Work out the finished part from the listing and answer in its coordinate system (mm). Face numbers are marked on the shaded views. Coordinates: 2 decimals unless noted, no trailing zeros. Order: outer loops, then holes, each group sorted by start corner. A loop starts at its lowest first (then second) coordinate and runs counter-clockwise, first axis right, second up. Notation, with made-up numbers: M 76.5,24 L 92.5,24 A18 ccw 92.5,50 Z; hole C 30.5,-34 d10. An arc over 180 degrees is marked long. Answer in a Markdown table with one row per item. Add a question column.
Item 1: The part is cut by section C-C (y = 1.9). Write down the section's boundary in (x, z).
Item 2: The part is cut by section B-B (x = -2.4). Write down the section's boundary in (y, z), then the cut area to 3 significant figures.
Item 3: Consider line 1 (Y direction, x = 0.1, z = 6.25); line 2 (Y direction, x = -0.85, z = 16.75); line 3 (X direction, y = 0.75, z = 5.75). Determine where each line is inside the solid, lowest interval first. Write a range as from..to.
Item 4: Flat-ended cylindrical pins translate along their axes: pin 1 Ø2 at (x, z) = (2, 13.5) entering from -Y; pin 2 Ø1.5 at (x, y) = (0, 0) entering from -Z; pin 3 Ø1 at (y, z) = (-2, 8) entering from -X. Find the tip coordinate at first contact, or state that the pin passes through.
Item 5: The mould has two halves that part along Y. Classify the marked faces 1, 2, 3 and 4: released by +Y, released by -Y, zero draft, split by the parting line, or undercut.
Item 6: The part is cut by section A-A (z = 4). Write down the section's boundary in (x, y).
Autodesk Inventor part; units mm, degrees
ref_plane "YZ Plane" through (0, 0, 0) normal (1, 0, 0) x (0, 1, 0)
ref_plane "XZ Plane" through (0, 0, 0) normal (0, 1, 0) x (-1, 0, 0)
ref_plane "XY Plane" through (0, 0, 0) normal (0, 0, 1) x (1, 0, 0)
sketch "スケッチ1" plane through (0, 0, 0) normal (0, 0, 1) x (1, 0, 0)
  circle A0 centre (0, 0) radius 3
  dimension "d0" = 6
extrude "押し出し1" add sketch "スケッチ1" along normal blind 20
sketch "スケッチ2" plane through (0, 0, 20) normal (0, 0, 1) x (1, 0, 0)
  point P0 (0, 0)
  point P1 (0, 0)
hole "穴1" at (0, 0, 20) direction (0, 0, -1) diameter 2.459 depth 8.8 tip angle 118
sketch "スケッチ3" plane through (0, 0, 0) normal (0, 0, -1) x (-1, 0, 0)
  circle A0 centre (0, 0) radius 1.2295
hole "穴2" at (0, 0, 0) direction (0, 0, 1) diameter 2.459 depth 8.8 tip angle 118
properties part number "base_part1" material "アルミニウム 6061"
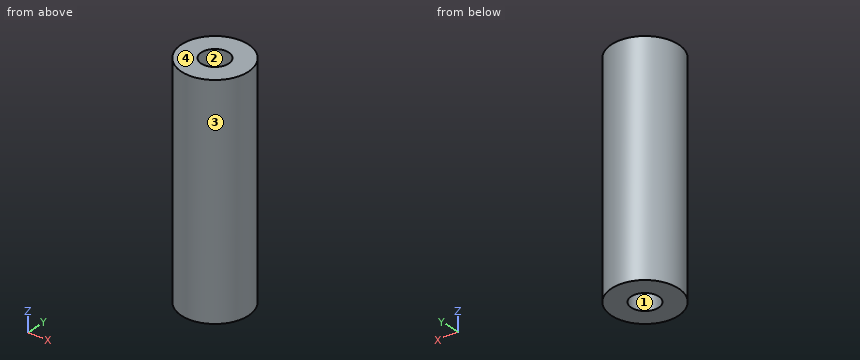
Reply:
| question | item | result |
|---|---|---|
| 1 | outline | M -2.32,0 L 2.32,0 L 2.32,20 L -2.32,20 Z |
| 2 | outline | M -1.8,0 L 1.8,0 L 1.8,20 L -1.8,20 Z |
| 2 | area | 72.0 mm2 |
| 3 | line 1 | y = -3..-1.23, 1.23..3 |
| 3 | line 2 | y = -2.88..-0.89, 0.89..2.88 |
| 3 | line 3 | x = -2.9..-0.97, 0.97..2.9 |
| 4 | pin 1 | stops at y = -2.83 |
| 4 | pin 2 | stops at z = 9.09 |
| 4 | pin 3 | stops at x = -2.6 |
| 5 | face 1 | undercut |
| 5 | face 2 | undercut |
| 5 | face 3 | split by the parting line |
| 5 | face 4 | zero draft |
| 6 | outline | C 0,0 d6; hole C 0,0 d2.46 |
